```python
from build123d import *

# Parameters (mm, degrees)
F0_W = 1
F0_H = 1


with BuildPart() as f1:
    # F0 (on Top) → F1 (revolve)
    with BuildSketch(Plane.XY):
        with BuildLine():
            Line((36, -22.526782), (36, -27.526782))
            Line((36, -27.526782), (38, -27.526782))
            ThreePointArc((38, -27.526782), (38.707107, -27.233889), (39, -26.526782))
            Line((39, -26.526782), (39, -21.526782))
            Line((39, -21.526782), (37, -21.526782))
            ThreePointArc((37, -21.526782), (36.292893, -21.819675), (36, -22.526782))
        make_face()
        Polygon((37, -19.526782), (37, -21.526782), (39, -21.526782), (39, -19.526782), (38, -19.526782), align=None)
        with Locations((37.5, -19.026782)):
            Rectangle(F0_W, F0_H)
        Polygon((37, -16.526782), (37, -18.526782), (38, -18.526782), (39, -18.526782), (39, -16.526782), (38, -16.526782), align=None)
        with Locations((37.5, -16.026782)):
            Rectangle(F0_W, F0_H)
        Polygon((37, -13.526782), (37, -15.526782), (38, -15.526782), (39, -15.526782), (39, -13.526782), align=None)
        with BuildLine():
            ThreePointArc((36, -12.526782), (36.292893, -13.233889), (37, -13.526782))
            Line((37, -13.526782), (39, -13.526782))
            Line((39, -13.526782), (39, -8.526782))
            ThreePointArc((39, -8.526782), (38.707107, -7.819675), (38, -7.526782))
            Line((38, -7.526782), (37, -7.526782))
            ThreePointArc((37, -7.526782), (36.292893, -7.819675), (36, -8.526782))
            Line((36, -8.526782), (36, -12.526782))
        make_face()
    revolve(axis=Axis((32, -17.526782, 0), (0, 1, 0)))


with BuildPart() as f1_1:
    # F2: moved
    add(f1.part.moved(Location((0, -2, 0))))


solid = f1_1.part
```
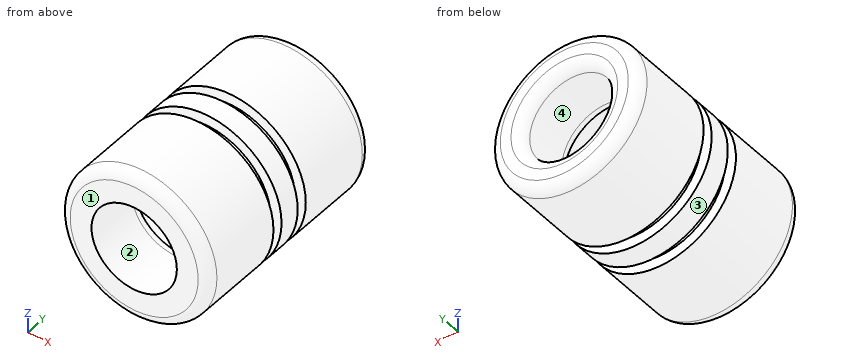
Input: part model. Units: mm. Frame: model coordinates. Face numbers are marked on the shaded views. Coordinates: 2 decimals unless noted, no trailing zeros. Loops run counter-clockwise (first coordinate to the right, second up) from the corner with the lowest first, then second, coordinate; pieces in that order, holes last. Notation, with made-up numbers: (6, 7.25) - (40, 7.25) arc R25 ccw to (40, 37.25) - close; hole circle Ø5 at (-14.75, 3). An arc over 180 degrees is marked (long way). Answer in a Markdown table with one row per item.
(1) Cut plane B-B on y = -13.25. Output: boundary loops of the cut face in (x, z).
Model answer:
| item | result |
|---|---|
| outline | circle Ø14 at (32, 0); hole circle Ø8 at (32, 0) |
(2) Cut plane A-A on y = -21. Output: boundary loops of the cut face in (x, z), plus the area to 3 significant figures.
Model answer:
| item | result |
|---|---|
| outline | circle Ø12 at (32, 0); hole circle Ø10 at (32, 0) |
| area | 34.6 mm² |
(3) Material intervals for L1, parallel to Z at x = 32, y = -19.75; L2, parallel to Z at x = 32, y = -11.9; L3, parallel to X at y = -13.2, z = 0, sorted ascending. Write a range as from..to.
Model answer:
| item | result |
|---|---|
| L1 | z = -7..-5, 5..7 |
| L2 | z = -7..-4, 4..7 |
| L3 | x = 25..28, 36..39 |
(4) Mould query, pull axis Z, two halves, no side actions, for the marked faces 1, 2, 3 and 4. Classes: pulls with the +Z half, pulls with the -Z half, needs draft (parallel to the pull), parting line crosses it, or undercut.
Model answer:
| item | result |
|---|---|
| face 1 | needs draft |
| face 2 | undercut |
| face 3 | parting line crosses it |
| face 4 | undercut |
(5) Pin query (flat end, axial travel): P1, Ø1.5, axis at x = 35, y = -13.5, coming from the +Z side; P2, Ø5, axis at x = 35.5, y = -18, coming from the -Z side; P3, Ø1.5, axis at y = -16, z = 1, coming from the +X side. Return the tip coordinate at first contact, or that it passes through.
Model answer:
| item | result |
|---|---|
| P1 | stops at z = 6.63 |
| P2 | stops at z = -6.92 |
| P3 | stops at x = 39 |
